The model under review builds one solid part; all positions refer to its coordinate system, in mm. A direction names the side the tool comes from. Round coordinates to 2 decimals unless told otherwise and drop trailing zeros. Write each loop counter-clockwise with the first axis right and the second up, starting at its lowest first coordinate (ties: lowest second). Pieces come first, ordered by that corner, then holes. Notation, with made-up numbers: M -15.75,21 L 14.25,21 A33 cw 14.25,60 Z; hole C -9,45 d5. An arc over 180 degrees is marked long. One line per item, written item: value. Start each with the question number.
1) Tool access review of faces 1 (the face through (-61.69, -1.13, -29.84)), 2 (the face through (-24, -1, -16.256)): name each direction out of +Z, -Z, +X, -X, +Y, -Y from which nothing blocks a thin tool from reaching the whole face with its end or side.
2) Take a section at A-A, the plane z = 8.5. Write out the cut boundary in (x, y).
3) For P1, Ø4.5, axis at x = 57.15, z = 25.4, coming from the -Y side; P2, Ø4.5, axis at x = -57.15, z = -25.4, coming from the +Y side, all flat-tipped, find the tip position at first contact; note any pin that passes through.
4) Mouldability with a two-part tool opening along Z and no side actions: class faces 3 (the face through (-1, 0, 0)), 4 (the face through (61.59, -1.13, -29.94)), 5 (the face through (-55.333, -1.127, -24.828)), 6 (the face through (1, -1, 31.75)) as +Z half, -Z half, draft (parallel to the pull), parting line (faces both ways), or undercut.
5) Wall thickness on probe 1 along X at (y, z) = (-0.2, -10); probe 2 along Z at (x, y) = (-57.15, -0.8) (3 decimals); probe 3 along X at (y, z) = (-2.65, -12): over which ranges is each line inside the solid? List them lowest first.
6) Take a section at B-B, the plane x = -23.5. Write out the cut boundary in (y, z).
from build123d import *

# Parameters (mm, degrees)
F0_R     = 1.905
F1_DEPTH = 3.81
F2_R     = 1.524
F3_SIZE  = 1.524


with BuildPart() as f1:
    # F0 (on Front) → F1 (new body)
    with BuildSketch(Plane.XZ):
        with BuildLine():
            ThreePointArc((63.5, 25.4), (61.640128, 29.890128), (57.15, 31.75))
            Line((57.15, 31.75), (-57.15, 31.75))
            ThreePointArc((-57.15, 31.75), (-61.640128, 29.890128), (-63.5, 25.4))
            Line((-63.5, 25.4), (-63.5, -25.4))
            ThreePointArc((-63.5, -25.4), (-61.640128, -29.890128), (-57.15, -31.75))
            Line((-57.15, -31.75), (57.15, -31.75))
            ThreePointArc((57.15, -31.75), (61.640128, -29.890128), (63.5, -25.4))
            Line((63.5, -25.4), (63.5, 25.4))
        make_face()
        with Locations((-57.15, -25.4)):
            Circle(F0_R, mode=Mode.SUBTRACT)
        with Locations((57.15, -25.4)):
            Circle(F0_R, mode=Mode.SUBTRACT)
        with BuildLine():
            ThreePointArc((-38.989, 14.986), (-38.617026, 15.884026), (-37.719, 16.256))
            Line((-37.719, 16.256), (-11.43, 16.256))
            ThreePointArc((-11.43, 16.256), (-10.531974, 15.884026), (-10.16, 14.986))
            Line((-10.16, 14.986), (-10.16, -14.986))
            ThreePointArc((-10.16, -14.986), (-10.531974, -15.884026), (-11.43, -16.256))
            Line((-11.43, -16.256), (-37.719, -16.256))
            ThreePointArc((-37.719, -16.256), (-38.617026, -15.884026), (-38.989, -14.986))
            Line((-38.989, -14.986), (-38.989, 14.986))
        make_face(mode=Mode.SUBTRACT)
        with Locations((-57.15, 25.4)):
            Circle(F0_R, mode=Mode.SUBTRACT)
        with BuildLine():
            ThreePointArc((10.16, 14.986), (10.531974, 15.884026), (11.43, 16.256))
            Line((11.43, 16.256), (37.719, 16.256))
            ThreePointArc((37.719, 16.256), (38.617026, 15.884026), (38.989, 14.986))
            Line((38.989, 14.986), (38.989, -14.986))
            ThreePointArc((38.989, -14.986), (38.617026, -15.884026), (37.719, -16.256))
            Line((37.719, -16.256), (11.43, -16.256))
            ThreePointArc((11.43, -16.256), (10.531974, -15.884026), (10.16, -14.986))
            Line((10.16, -14.986), (10.16, 14.986))
        make_face(mode=Mode.SUBTRACT)
        with Locations((57.15, 25.4)):
            Circle(F0_R, mode=Mode.SUBTRACT)
    extrude(amount=F1_DEPTH)

    # F2
    f2_edges = [f1.edges().sort_by_distance(p)[0] for p in [
        (-38.989, -3.81, 0),
        (10.16, -3.81, 0),
        (-63.5, -3.81, 0),
    ]]
    fillet(f2_edges, radius=F2_R)

    # F3
    f3_edges = [f1.edges().sort_by_distance(p)[0] for p in [
        (-59.055, -3.81, 25.4),
        (-59.055, -3.81, -25.4),
        (55.245, -3.81, -25.4),
        (55.245, -3.81, 25.4),
    ]]
    chamfer(f3_edges, length=F3_SIZE)


solid = f1.part
Checked values:
1. face 1: -Z, -X, +Y, -Y
1. face 2: +Y, -Y
2. outline: M -63.5,-2.29 A1.52 ccw -61.98,-3.81 L -40.51,-3.81 A1.52 ccw -38.99,-2.29 L -38.99,0 L -63.5,0 Z; M -10.16,-2.29 A1.52 ccw -8.64,-3.81 L 8.64,-3.81 A1.52 ccw 10.16,-2.29 L 10.16,0 L -10.16,0 Z; M 38.99,-2.29 A1.52 ccw 40.51,-3.81 L 61.98,-3.81 A1.52 ccw 63.5,-2.29 L 63.5,0 L 38.99,0 Z
3. P1: stops at y = -2.63
3. P2: stops at y = 0
4. face 3: draft
4. face 4: -Z half
4. face 5: undercut
4. face 6: +Z half
5. probe 1: x = -63.5 to -38.99, -10.16 to 10.16, 38.99 to 63.5
5. probe 2: z = -31.75 to -27.305, -23.495 to 23.495, 27.305 to 31.75
5. probe 3: x = -63.46 to -39.03, -10.12 to 10.12, 39.03 to 63.46
6. outline: M -3.81,-30.23 A1.52 ccw -2.29,-31.75 L 0,-31.75 L 0,-16.26 L -2.29,-16.26 A1.52 ccw -3.81,-17.78 Z; M -3.81,17.78 A1.52 ccw -2.29,16.26 L 0,16.26 L 0,31.75 L -2.29,31.75 A1.52 ccw -3.81,30.23 Z
